Work out the finished part from the listing and answer in its coordinate system (mm). Face numbers are marked on the shaded views. A direction names the side the tool comes from. Coordinates: 2 decimals unless noted, no trailing zeros. Loops run counter-clockwise (first coordinate to the right, second up) from the corner with the lowest first, then second, coordinate; pieces in that order, holes last. Notation, with made-up numbers: (-7.5, 68.25) -> (39.5, 68.25) arc R24 cw to (39.5, 100.25) -> close; hole circle Ø6 at (10.25, 82). An arc over 180 degrees is marked (long way). Use a Markdown table: item, result.
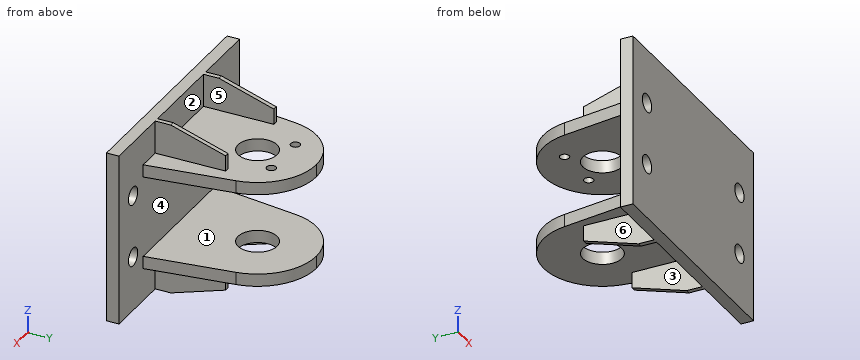
from build123d import *

# Parameters (mm, degrees)
SKETCH_1_W                  = 300
SKETCH_1_H                  = 220
EXTRUDE_1_DEPTH             = 16
SKETCH_2_R                  = 11.5
CUT_EXTRUDE_1_DEPTH         = 373.365411928
PATTERN_LINEAR_1_COUNT      = 2
PATTERN_LINEAR_1_PITCH      = 230
PATTERN_LINEAR_1_COUNT_DIR2 = 2
PATTERN_LINEAR_1_PITCH_DIR2 = 80
SKETCH_3_W                  = 180
SKETCH_3_H                  = 16
EXTRUDE_2_DEPTH             = 175
CUT_EXTRUDE_2_DEPTH         = 398.699635403
CUT_EXTRUDE_3_DEPTH         = 398.699635403
SKETCH_8_R                  = 25
CUT_EXTRUDE_4_DEPTH         = 398.699635403
PATTERN_LINEAR_3_COUNT      = 2
PATTERN_LINEAR_3_PITCH      = 120
SKETCH_9_R                  = 6
CUT_EXTRUDE_5_DEPTH         = 16
PATTERN_LINEAR_4_COUNT      = 2
PATTERN_LINEAR_4_PITCH      = 60
SKETCH_10_W                 = 6
SKETCH_10_H                 = 42
EXTRUDE_3_DEPTH             = 90
PATTERN_LINEAR_5_COUNT      = 2
PATTERN_LINEAR_5_PITCH      = 120
PATTERN_LINEAR_5_COUNT_DIR2 = 2
PATTERN_LINEAR_5_PITCH_DIR2 = 178
CUT_EXTRUDE_6_DEPTH         = 363.680299989


with BuildPart() as part:
    # 草图1 → 凸台-拉伸1 (new body)
    with BuildSketch(Plane(origin=(0, 0, 0), x_dir=(1, 0, 0), z_dir=(0, 1, 0))):
        with Locations((150, 110)):
            Rectangle(SKETCH_1_W, SKETCH_1_H)
    extrude(amount=EXTRUDE_1_DEPTH)

    # 草图2 → 切除-拉伸1 (cut, through all)
    with BuildSketch(Plane(origin=(0, 16, 0), x_dir=(1, 0, 0), z_dir=(0, 1, 0))):
        with Locations(Location((35, 150, 0), (0, 0, 270))):
            Circle(SKETCH_2_R)
    cut_extrude_1 = extrude(amount=-CUT_EXTRUDE_1_DEPTH, mode=Mode.SUBTRACT)

    # 阵列(线性)1: Cut-Extrude 1 2 × 2
    with Locations(*[(i * PATTERN_LINEAR_1_PITCH, 0, j * PATTERN_LINEAR_1_PITCH_DIR2) for i in range(PATTERN_LINEAR_1_COUNT) for j in range(PATTERN_LINEAR_1_COUNT_DIR2) if (i, j) != (0, 0)]):
        add(cut_extrude_1, mode=Mode.SUBTRACT)

    # 草图3 → 凸台-拉伸2 (add)
    with BuildSketch(Plane(origin=(0, 16, 0), x_dir=(1, 0, 0), z_dir=(0, 1, 0))):
        with Locations((150, 170)):
            Rectangle(SKETCH_3_W, SKETCH_3_H)
    extrude_2 = extrude(amount=EXTRUDE_2_DEPTH)

    # 草图5 → 切除-拉伸2 (cut, through all)
    with BuildSketch(Plane(origin=(0, 0, -178), x_dir=(-1, 0, 0), z_dir=(0, 0, -1))):
        with BuildLine():
            Line((-60, 16), (-75.749362078, 126.57557413))
            ThreePointArc((-75.749362078, 126.57557413), (-100.848031879, 172.648777832), (-150, 191))
            Line((-150, 191), (-60, 191))
            Line((-60, 191), (-60, 16))
        make_face()
    cut_extrude_2 = extrude(amount=-CUT_EXTRUDE_2_DEPTH, mode=Mode.SUBTRACT)

    # 草图7 → 切除-拉伸3 (cut, through all)
    with BuildSketch(Plane(origin=(0, 0, -178), x_dir=(-1, 0, 0), z_dir=(0, 0, -1))):
        with BuildLine():
            Line((-224.250637922, 126.57557413), (-240, 16))
            Line((-240, 16), (-240, 191))
            Line((-240, 191), (-150, 191))
            ThreePointArc((-150, 191), (-199.151968121, 172.648777832), (-224.250637922, 126.57557413))
        make_face()
    cut_extrude_3 = extrude(amount=-CUT_EXTRUDE_3_DEPTH, mode=Mode.SUBTRACT)

    # 草图8 → 切除-拉伸4 (cut, through all)
    with BuildSketch(Plane(origin=(0, 0, -178), x_dir=(-1, 0, 0), z_dir=(0, 0, -1))):
        with Locations((-150, 116)):
            Circle(SKETCH_8_R)
    cut_extrude_4 = extrude(amount=-CUT_EXTRUDE_4_DEPTH, mode=Mode.SUBTRACT)

    # 阵列(线性)3: 凸台-拉伸2, 切除-拉伸2, 切除-拉伸3, 切除-拉伸4 ×2
    with Locations(*[(0, 0, i * PATTERN_LINEAR_3_PITCH) for i in range(1, PATTERN_LINEAR_3_COUNT)]):
        add(extrude_2)
        add(cut_extrude_2, mode=Mode.SUBTRACT)
        add(cut_extrude_3, mode=Mode.SUBTRACT)
        add(cut_extrude_4, mode=Mode.SUBTRACT)

    # 草图9 → 切除-拉伸5 (cut)
    with BuildSketch(Plane.XY.offset(-42)):
        with Locations((120, 149)):
            Circle(SKETCH_9_R)
    cut_extrude_5 = extrude(amount=-CUT_EXTRUDE_5_DEPTH, mode=Mode.SUBTRACT)

    # 阵列(线性)4: 切除-拉伸5 ×2
    with Locations(*[(i * PATTERN_LINEAR_4_PITCH, 0, 0) for i in range(1, PATTERN_LINEAR_4_COUNT)]):
        add(cut_extrude_5, mode=Mode.SUBTRACT)

    # 草图10 → 凸台-拉伸3 (add)
    with BuildSketch(Plane(origin=(0, 16, 0), x_dir=(1, 0, 0), z_dir=(0, 1, 0))):
        with Locations((87, 21)):
            Rectangle(SKETCH_10_W, SKETCH_10_H)
    extrude_3 = extrude(amount=EXTRUDE_3_DEPTH)

    # 阵列(线性)5: Extrude 3 2 × 2
    with Locations(*[(i * PATTERN_LINEAR_5_PITCH, 0, -j * PATTERN_LINEAR_5_PITCH_DIR2) for i in range(PATTERN_LINEAR_5_COUNT) for j in range(PATTERN_LINEAR_5_COUNT_DIR2) if (i, j) != (0, 0)]):
        add(extrude_3)

    # 草图11 → 切除-拉伸6 (cut, through all)
    with BuildSketch(Plane.ZY.offset(-84)):
        Polygon((0, 106), (-22, 106), (0, 36), align=None)
        Polygon((-220, 106), (-220, 36), (-198, 106), align=None)
    extrude(amount=-CUT_EXTRUDE_6_DEPTH, mode=Mode.SUBTRACT)


solid = part.part
Q1. Section A-A on x = 120 is taken. Determine the outline of the cut face in (y, z).
Solved:
| item | result |
|---|---|
| outline | (0, -220) -> (16, -220) -> (16, -178) -> (184.74, -178) -> (184.74, -162) -> (16, -162) -> (16, -58) -> (143, -58) -> (143, -42) -> (16, -42) -> (16, 0) -> (0, 0) -> close; (155, -58) -> (184.74, -58) -> (184.74, -42) -> (155, -42) -> close |
Q2. Consider line 1 (Y direction, x = 150, z = -47.75); line 2 (Z direction, x = 143.5, y = 183.5); line 3 (Y direction, x = 259, z = -32). Determine where each line is inside the solid, lowest interval first. Write a range as [from, to].
Solved:
| item | result |
|---|---|
| line 1 | [0, 91], [141, 191] |
| line 2 | [-178, -162], [-58, -42] |
| line 3 | [0, 16] |
Q3. Given pin 1 Ø3 at (x, z) = (151.5, -110) entering from +Y; pin 2 Ø21 at (y, z) = (41.5, -200) entering from +X; pin 3 Ø12 at (y, z) = (91.5, -174.5) entering from +X; pin 4 Ø20.5 at (x, z) = (35, -150) entering from -Y, each flat-ended and moving along its own axis, determine where each tip first touches the part or whether it passes through.
Solved:
| item | result |
|---|---|
| pin 1 | y = 16 |
| pin 2 | x = 210 |
| pin 3 | x = 230.1 |
| pin 4 | through |
Q4. Section B-B on z = -51 is taken. Determine the outline of the cut face in (x, y), and give its area (3 significant figures).
Solved:
| item | result |
|---|---|
| outline | (0, 0) -> (300, 0) -> (300, 16) -> (240, 16) -> (224.25, 126.58) arc R75 ccw to (75.75, 126.58) -> (60, 16) -> (0, 16) -> close; hole circle Ø12 at (120, 149); hole circle Ø50 at (150, 116); hole circle Ø12 at (180, 149) |
| area | 28,000 mm² |
Q5. Determine the mould class of the marked faces 1 and 2 for opening direction Z: pulls with the +Z half, pulls with the -Z half, needs draft (parallel to the pull), parting line crosses it, or undercut.
Solved:
| item | result |
|---|---|
| face 1 | undercut |
| face 2 | needs draft |
Q6. For the marked faces 3, 4, 5 and 6, determine the directions among +Z, -Z, +X, -X, +Y, -Y from which every point of the face is accessible in a straight line to the end or side of a thin tool.
Solved:
| item | result |
|---|---|
| face 3 | -Z, +Y |
| face 4 | +Y |
| face 5 | +Z, +Y |
| face 6 | -Z, -X, +Y |
Q7. Section D-D on y = 116 is taken. Determine the outline of the cut face in (x, z), and give its area (3 significant figures).
Solved:
| item | result |
|---|---|
| outline | (74.24, -178) -> (125, -178) -> (125, -162) -> (74.24, -162) -> close; (74.24, -58) -> (125, -58) -> (125, -42) -> (74.24, -42) -> close; (175, -178) -> (225.76, -178) -> (225.76, -162) -> (175, -162) -> close; (175, -58) -> (225.76, -58) -> (225.76, -42) -> (175, -42) -> close |
| area | 3,250 mm² |
Q8. Section C-C on y = 19.5 is taken. Determine the outline of the cut face in (x, z), and give its area (3 significant figures).
Solved:
| item | result |
|---|---|
| outline | (60.5, -178) -> (84, -178) -> (84, -220) -> (90, -220) -> (90, -178) -> (204, -178) -> (204, -220) -> (210, -220) -> (210, -178) -> (239.5, -178) -> (239.5, -162) -> (60.5, -162) -> close; (60.5, -58) -> (239.5, -58) -> (239.5, -42) -> (210, -42) -> (210, 0) -> (204, 0) -> (204, -42) -> (90, -42) -> (90, 0) -> (84, 0) -> (84, -42) -> (60.5, -42) -> close |
| area | 6,740 mm² |
